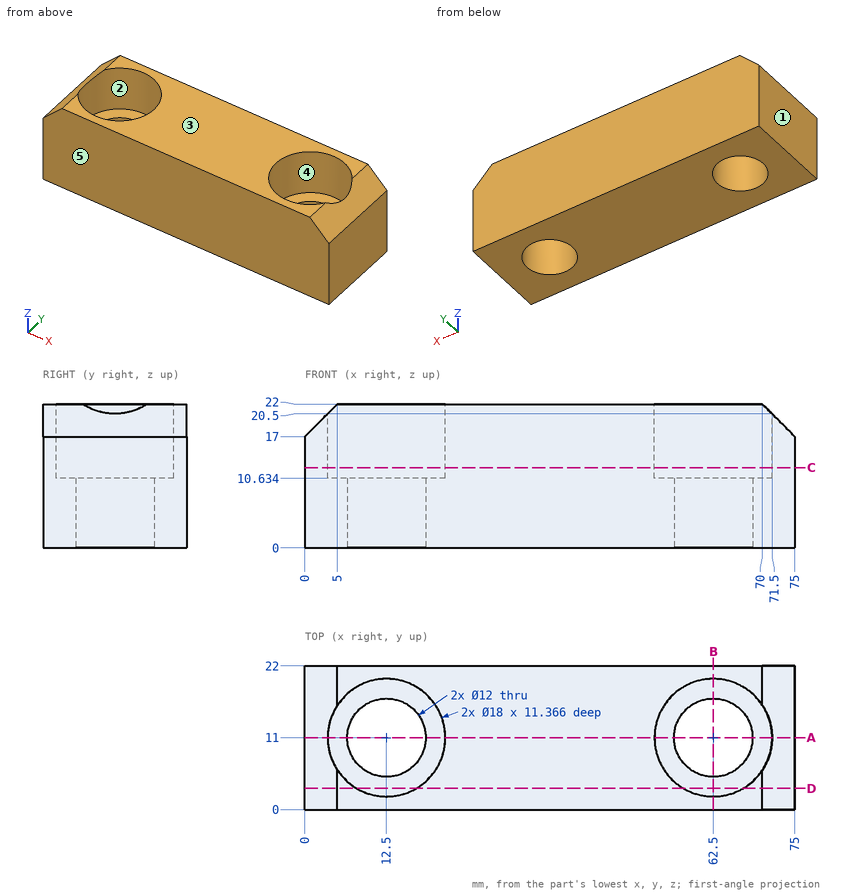
Design review of the part shown in the three views and the two pictorial views. Dimensions are in mm from the part's minimum x, y and z. A direction names the side the tool comes from. Round coordinates to 2 decimals unless told otherwise and drop trailing zeros. Write each loop counter-clockwise with the first axis right and the second up, starting at its lowest first coordinate (ties: lowest second). Pieces come first, ordered by that corner, then holes. Notation, with made-up numbers: M -39,11.5 L -31,11.5 A30 ccw -31,39.5 Z; hole C -20.5,13 d11. An arc over 180 degrees is marked long. One line per item, written item: value. Start each with the question number.
1. Clearance check with flat-ended pins moving along their axes: P1, Ø5, axis at x = 21, z = 9.5, coming from the -Y side; P2, Ø9, axis at x = 16, y = 9.5, coming from the +Z side. State where each tip first meets the part, or that it passes through.
2. Take a section at D-D on y = 3.25. State the section outline as (x, z) points.
3. Take a section at A-A on y = 11. State the section outline as (x, z) points.
4. Draft analysis for pull direction X (two halves, no side actions). For the marked faces 1, 2 and 3, state which applies: pulls with the +X half, pulls with the -X half, needs draft (parallel to the pull), parting line crosses it, or undercut.
5. To check wall thickness, follow probe 1 along X at (y, z) = (11, 15.25); probe 2 along X at (y, z) = (17, 18.5); probe 3 along Y at (x, z) = (12.5, 8.25). State the ranges of each line that lie inside material, in increasing order. Write a range as from..to.
6. For the marked faces 4 and 5, list the 3-axis set-ups (+Z, -Z, +X, -X, +Y, -Y) from which the entire face can be reached by the end or side of a thin tool; tool diameter is ignored.
7. Take a section at B-B on x = 62.5. State the section outline as (y, z) points, then the cut area to 3 significant figures.
8. Take a section at C-C on z = 12.25. State the section outline as (x, y) points, then the cut area to 3 significant figures.
Computed:
1. P1: stops at y = 0
1. P2: stops at z = 10.63
2. outline: M 0,0 L 75,0 L 75,17 L 70,22 L 67.08,22 L 67.08,10.63 L 57.92,10.63 L 57.92,22 L 17.08,22 L 17.08,10.63 L 7.92,10.63 L 7.92,22 L 5,22 L 0,17 Z
3. outline: M 0,0 L 6.5,0 L 6.5,10.63 L 3.5,10.63 L 3.5,20.5 L 0,17 Z; M 18.5,0 L 56.5,0 L 56.5,10.63 L 53.5,10.63 L 53.5,22 L 21.5,22 L 21.5,10.63 L 18.5,10.63 Z; M 68.5,0 L 75,0 L 75,17 L 71.5,20.5 L 71.5,10.63 L 68.5,10.63 Z
4. face 1: pulls with the -X half
4. face 2: undercut
4. face 3: needs draft
5. probe 1: x = 0..3.5, 21.5..53.5, 71.5..75
5. probe 2: x = 1.5..5.79, 19.21..55.79, 69.21..73.5
5. probe 3: y = 0..5, 17..22
6. face 4: +Z
6. face 5: +Z, -Z, +X, -X, -Y
7. outline: M 0,0 L 5,0 L 5,10.63 L 2,10.63 L 2,22 L 0,22 Z; M 17,0 L 22,0 L 22,22 L 20,22 L 20,10.63 L 17,10.63 Z
7. area: 152 mm²
8. outline: M 0,0 L 75,0 L 75,22 L 0,22 Z; hole C 12.5,11 d18; hole C 62.5,11 d18
8. area: 1,140 mm²
